Here's how the part is built. I have some questions about the finished solid (model axes, mm). A direction names the side the tool comes from. Coordinates: 2 decimals unless noted, no trailing zeros. Write each loop counter-clockwise with the first axis right and the second up, starting at its lowest first coordinate (ties: lowest second). Pieces come first, ordered by that corner, then holes.
Item 1: For faces 4 (the face through (-28.5, 0, 5)), 5 (the face through (2.6, -0.3, 7.4)), 6 (the face through (0, 0, 2.3)), which set-ups out of +Z, -Z, +X, -X, +Y, -Y let a thin tool reach every point of the face, with its end or its side?
Item 2: I want a section at D-D (x = -22.5). Please give me the cut outline in (y, z).
Item 3: If we mould it in two halves opening along X, with no side actions, what happens to faces 1 (the face through (28.5, 0, 5)), 2 (the face through (-9, 0, 10)), 3 (the face through (-20.9, -0.3, 7.4))? For each: pulls with the +X half, pulls with the -X half, needs draft (parallel to the pull), parting line crosses it, or undercut.
Item 4: I'm going to push flat-ended pins straight in: P1, Ø3, axis at x = 3.5, y = -1.5, coming from the -Z side; P2, Ø4, axis at x = 15, y = -18.5, coming from the +Z side. Where does each tip first touch, or does it pass through?
Item 5: I want a section at C-C (x = -15.5). Please give me the cut outline in (y, z), and give its area (3 significant figures).
Item 6: I want a section at A-A (z = 8.25). Please give me the cut outline in (x, y), and give its area (3 significant figures).
Item 7: Please list where these lines run through material, in increasing order: line 1 (Z direction, x = -11, y = -19.5); line 2 (X direction, y = -3, z = 7.25); line 3 (Z direction, x = 18, y = 5).
from build123d import *

# Parameters (mm, degrees)
F1_DEPTH = 24
F3_W     = 10.4
F3_H     = 48
F4_DEPTH = 5.2
F5_SIZE  = 5.19999


# Not quite as in the source:
# - a fillet or chamfer is up to 0.001 mm smaller than in the source, because OpenCascade refuses the exact size


with BuildPart() as f1:
    # F0 (on Front) → F1 (new body, symmetric)
    with BuildSketch(Plane.XZ):
        Polygon((-28.5, 10), (-28.5, 0), (-26, 0), (-24, 2.3), (24, 2.3), (26, 0), (28.5, 0), (28.5, 10), align=None)
    extrude(amount=F1_DEPTH, both=True)

    # F3 (on offset) → F4 (cut)
    with BuildSketch(Plane.XY.offset(10)):
        with Locations((-18.3, 0)):
            Rectangle(F3_W, F3_H)
        Rectangle(F3_W, F3_H)
        with Locations((18.3, 0)):
            Rectangle(F3_W, F3_H)
    extrude(amount=-F4_DEPTH, mode=Mode.SUBTRACT)

    # F5 (size 5.2 in the source; OpenCascade refuses exactly that, so slightly less here)
    f5_edges = [f1.edges().sort_by_distance(p)[0] for p in [
        (-13.1, 0, 4.8),
        (-23.5, 0, 4.8),
        (-5.2, 0, 4.8),
        (5.2, 0, 4.8),
        (13.1, 0, 4.8),
        (23.5, 0, 4.8),
    ]]
    chamfer(f5_edges, length=F5_SIZE)


solid = f1.part
Answer:
1. face 4: +Z, -Z, -X, +Y, -Y
1. face 5: +Z, +Y, -Y
1. face 6: -Z, +Y, -Y
2. outline: (-24, 2.3) - (24, 2.3) - (24, 9) - (-24, 9) - close
3. face 1: pulls with the +X half
3. face 2: needs draft
3. face 3: undercut
4. P1: stops at z = 2.3
4. P2: stops at z = 10
5. outline: (-24, 2.3) - (24, 2.3) - (24, 7.6) - (-24, 7.6) - close
5. area: 254 mm2
6. outline: (-28.5, -24) - (-21.75, -24) - (-21.75, 24) - (-28.5, 24) - close; (-14.85, -24) - (-3.45, -24) - (-3.45, 24) - (-14.85, 24) - close; (3.45, -24) - (14.85, -24) - (14.85, 24) - (3.45, 24) - close; (21.75, -24) - (28.5, -24) - (28.5, 24) - (21.75, 24) - close
6. area: 1,740 mm2
7. line 1: z = 2.3 to 10
7. line 2: x = -28.5 to -20.75, -15.85 to -2.45, 2.45 to 15.85, 20.75 to 28.5
7. line 3: z = 2.3 to 5.1
